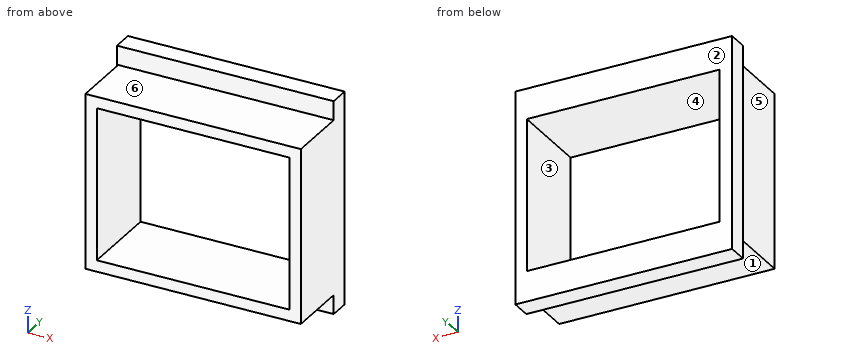
```python
from build123d import *

# Parameters (mm, degrees)
SKETCH_1_W      = 42.5
SKETCH_1_H      = 34.5
SKETCH_1_W_2    = 38
SKETCH_1_H_2    = 30
EXTRUDE_1_DEPTH = 12
SKETCH_2_W      = 42.75
SKETCH_2_H      = 42
SKETCH_2_W_2    = 38
SKETCH_2_H_2    = 30
EXTRUDE_2_DEPTH = 4


with BuildPart() as part:
    # Эскиз1 → Бобышка-Вытянуть1 (new body)
    with BuildSketch(Plane(origin=(0, 0, 0), x_dir=(1, 0, 0), z_dir=(0, 1, 0))):
        Rectangle(SKETCH_1_W, SKETCH_1_H)
        Rectangle(SKETCH_1_W_2, SKETCH_1_H_2, mode=Mode.SUBTRACT)
    extrude(amount=EXTRUDE_1_DEPTH)

    # Эскиз2 → Бобышка-Вытянуть2 (add)
    with BuildSketch(Plane(origin=(0, 12, 0), x_dir=(1, 0, 0), z_dir=(0, 1, 0))):
        with Locations((-0.125, 0)):
            Rectangle(SKETCH_2_W, SKETCH_2_H)
        Rectangle(SKETCH_2_W_2, SKETCH_2_H_2, mode=Mode.SUBTRACT)
    extrude(amount=EXTRUDE_2_DEPTH)


solid = part.part
```
For this review, take the finished solid that the model builds, in its own axes (mm). Face numbers are marked on the shaded views. A direction names the side the tool comes from. Give positions to 0.01 mm unless a question says otherwise; leave off trailing zeros. Write each loop counter-clockwise with the first axis right and the second up, starting at its lowest first coordinate (ties: lowest second). Pieces come first, ordered by that corner, then holes. Notation, with made-up numbers: M 66,28.25 L 97,28.25 A25 ccw 97,54.25 Z; hole C -36,21 d4. An arc over 180 degrees is marked long. Answer as a JSON object with one key per item and string values. Group by question number.
Item 1: Consider section C-C on z = 12.5. Write out the cut boundary in (x, y), plus the area to 3 significant figures.
Item 2: Consider section D-D on y = 13.25. Write out the cut boundary in (x, z), plus the area to 4 significant figures.
Item 3: For probe 1 along X at (y, z) = (7.5, -2); probe 2 along Z at (x, y) = (-14, 8.75); probe 3 along Z at (x, y) = (-5, 15.25), list the stretches that pass through material, from the lowest coordinate up. Write a range as [from, to].
Item 4: Draft analysis for pull direction X (two halves, no side actions). For the marked faces 4, 5 and 6, state which applies: +X half, -X half, draft (parallel to the pull), parting line (faces both ways), or undercut.
Item 5: For pin 1 Ø1 at (x, y) = (-6.5, 8) entering from +Z; pin 2 Ø8 at (x, y) = (7.5, 5.5) entering from -Z; pin 3 Ø2 at (y, z) = (10, -5) entering from -X, all flat-tipped, find the tip position at first contact; note any pin that passes through.
Item 6: Tool access review of the marked faces 1, 2 and 3: name each direction out of +Z, -Z, +X, -X, +Y, -Y from which nothing blocks a thin tool from reaching the whole face with its end or side.
Item 7: Consider section A-A on x = 16.5. Write out the cut boundary in (y, z).
Item 8: Consider section B-B on y = 8.75. Write out the cut boundary in (x, z).
Check result:
{
 "1": {"outline": "M -21.5,12 L -21.25,12 L -21.25,0 L -19,0 L -19,16 L -21.5,16 Z; M 19,0 L 21.25,0 L 21.25,16 L 19,16 Z", "area": "73.0 mm^2"},
 "2": {"outline": "M -21.5,-21 L 21.25,-21 L 21.25,21 L -21.5,21 Z; hole M -19,-15 L 19,-15 L 19,15 L -19,15 Z", "area": "655.5 mm^2"},
 "3": {"probe 1": "x = [-21.25, -19], [19, 21.25]", "probe 2": "z = [-17.25, -15], [15, 17.25]", "probe 3": "z = [-21, -15], [15, 21]"},
 "4": {"face 4": "undercut", "face 5": "-X half", "face 6": "draft"},
 "5": {"pin 1": "stops at z = 17.25", "pin 2": "stops at z = -17.25", "pin 3": "stops at x = -21.25"},
 "6": {"face 1": "-Z, +X, -X, -Y", "face 2": "+Z, -Z, +X, -X, +Y", "face 3": "+Y, -Y"},
 "7": {"outline": "M 0,-17.25 L 12,-17.25 L 12,-21 L 16,-21 L 16,-15 L 0,-15 Z; M 0,15 L 16,15 L 16,21 L 12,21 L 12,17.25 L 0,17.25 Z"},
 "8": {"outline": "M -21.25,-17.25 L 21.25,-17.25 L 21.25,17.25 L -21.25,17.25 Z; hole M -19,-15 L 19,-15 L 19,15 L -19,15 Z"}
}
